Check sheet for the modelled part. Datum: model origin and axes. Units: mm. Round coordinates to 2 decimals unless told otherwise and drop trailing zeros. Write each loop counter-clockwise with the first axis right and the second up, starting at its lowest first coordinate (ties: lowest second). Pieces come first, ordered by that corner, then holes. Notation, with made-up numbers: (51, 87.25) -> (95, 87.25) arc R19 ccw to (95, 91.25) -> close; hole circle Ø2 at (14.25, 19.5). An arc over 180 degrees is marked (long way). Write item = value, one per line.
from build123d import *

# Parameters (mm, degrees)
F1_DEPTH = 75


with BuildPart() as f1:
    # F0 (on Front) → F1 (new body)
    with BuildSketch(Plane.XZ):
        with BuildLine():
            ThreePointArc((233.020331, -56.316324), (11.13377, -103.106166), (-212.330451, -64.54871))
            Line((-212.330451, -64.54871), (-216.468156, -73.675685))
            ThreePointArc((-216.468156, -73.675685), (11.327825, -113.104287), (237.509549, -65.27698))
            Line((237.509549, -65.27698), (233.020331, -56.316324))
        make_face()
        with BuildLine():
            ThreePointArc((266.345782, -29.958453), (4.809679, -93.189537), (-257.718636, -34.213378))
            Line((-257.718636, -34.213378), (-262.368917, -43.072499))
            ThreePointArc((-262.368917, -43.072499), (-237.592465, -54.376272), (-212.330451, -64.54871))
            ThreePointArc((-212.330451, -64.54871), (11.13377, -103.106166), (233.020331, -56.316324))
            ThreePointArc((233.020331, -56.316324), (252.487762, -47.743164), (271.64038, -38.488046))
            Line((271.64038, -38.488046), (266.345782, -29.958453))
        make_face()
        with BuildLine():
            ThreePointArc((300, 0), (0, -83.209062), (-300, 0))
            Line((-300, 0), (-305.151002, -8.5713))
            ThreePointArc((-305.151002, -8.5713), (-281.726705, -21.932266), (-257.718636, -34.213378))
            ThreePointArc((-257.718636, -34.213378), (4.809679, -93.189537), (266.345782, -29.958453))
            ThreePointArc((266.345782, -29.958453), (285.948415, -19.627802), (305.151002, -8.5713))
            Line((305.151002, -8.5713), (300, 0))
        make_face()
    extrude(amount=F1_DEPTH)


solid = f1.part
(1) Material ranges on L1, parallel to X at y = -55.5, z = -35; L2, parallel to X at y = -24, z = -24; L3, parallel to Z at x = -80, y = -55.5, recorded low to high. Write a range as [from, to].
Worked answers:
L1 = [-258.13, -232.01], [232.01, 269.48]
L2 = [-277.87, -255.86], [255.86, 277.87]
L3 = [-107.96, -77.69]
(2) Sectioned sample at B-B on z = -19. Enter the section's corners in (x, y), then the cut area to 3 significant figures.
Worked answers:
outline = (-287.08, -75) -> (-265.84, -75) -> (-265.84, 0) -> (-287.08, 0) -> close; (265.84, -75) -> (287.08, -75) -> (287.08, 0) -> (265.84, 0) -> close
area = 3,190 mm²
(3) Go/stop test with flat-tipped pins: P1, Ø1.5, axis at x = -170, y = -35, coming from the -Z side; P2, Ø1, axis at y = -14.5, z = -13.5, coming from the +X side; P3, Ø6, axis at y = -25, z = -52.5, coming from the +X side. Record where each tip stops, or that it passes through.
Worked answers:
P1 = -89.36
P2 = 297.66
P3 = 248.65
(4) Sectioned sample at D-D on z = -92.5. Enter the section's corners in (x, y).
Worked answers:
outline = (-157.91, -75) -> (157.91, -75) -> (157.91, 0) -> (-157.91, 0) -> close
(5) Sectioned sample at A-A on y = -41.5. Enter the section's corners in (x, z).
Worked answers:
outline = (-305.15, -8.57) arc R592.41 ccw to (-257.72, -34.21) -> (-262.37, -43.07) arc R602.41 ccw to (-212.33, -64.55) -> (-216.47, -73.68) arc R612.41 ccw to (237.51, -65.28) -> (233.02, -56.32) arc R602.41 ccw to (271.64, -38.49) -> (266.35, -29.96) arc R592.41 ccw to (305.15, -8.57) -> (300, 0) arc R582.41 cw to (-300, 0) -> close
(6) Sectioned sample at C-C on x = 0. Enter the section's corners in (y, z).
Worked answers:
outline = (-75, -113.21) -> (0, -113.21) -> (0, -83.21) -> (-75, -83.21) -> close
(7) Release check for a two-part mould opening along X. For faces 1 (the cylindrical face through (4.412, -36.975, -83.192)), 2 (the cylindrical face through (-282.06, -36.98, -21.75)), 3 (the cylindrical face through (8.072, -36.975, -113.156)) record: pulls with the +X half, pulls with the -X half, needs draft (parallel to the pull), parting line crosses it, or undercut.
Worked answers:
face_1 = undercut
face_2 = pulls with the -X half
face_3 = parting line crosses it
